Here's how the part is built. I have some questions about the finished solid (model axes, mm). A direction names the side the tool comes from. Round coordinates to 2 decimals unless told otherwise and drop trailing zeros. Loops run counter-clockwise (first coordinate to the right, second up) from the corner with the lowest first, then second, coordinate; pieces in that order, holes last. Notation, with made-up numbers: M 79.25,72.25 L 106.25,72.25 A34 cw 106.25,109.25 Z; hole C 12.25,55.5 d9. An arc over 180 degrees is marked long. Use a Markdown table: item, result.
from build123d import *

# Parameters (mm, degrees)
BODYS_W                        = 48
BODYS_H                        = 114
BODY_DEPTH                     = 1.7
MIRROR1_START                  = -1.7
MIRROR1_OUTLINE_R              = 4.1
MIRROR1_DEPTH                  = 3.4
KNUCKLEBODY_REACH              = 63.87
KNUCKLEBODY_DIRECTION_2_REACH  = 63.87
KNUCKLECUT_DEPTH               = 71.965414111
KNUCKLECUT_DEPTH_BACK          = 71.965414111
KNUCKLECUTS_W                  = 17
KNUCKLECUTS_H                  = 22
HOLECHAMFER_SIZE               = 1.4
F_11_0_11_DIAMETER_HOLE2_D     = 11
F_11_0_11_DIAMETER_HOLE2_DEPTH = 4
F_11_0_11_DIAMETER_HOLE2_TIP   = 3.304733405


# Read off the part's stored shape, not the designer's step: Mirror1
with BuildPart() as part:
    # BodyS → Body (new, symmetric)
    with BuildSketch(Plane.XY):
        Rectangle(BODYS_W, BODYS_H)
    extrude(amount=BODY_DEPTH, both=True)

    # Mirror1 outline → Mirror1 (cut)
    with BuildSketch(Plane.XY.offset(MIRROR1_START)):
        with Locations((-14.5, 15.5)):
            Circle(MIRROR1_OUTLINE_R)
        with Locations((1.5, 44)):
            Circle(MIRROR1_OUTLINE_R)
        with Locations((-14.5, -15.5)):
            Circle(MIRROR1_OUTLINE_R)
        with Locations((1.5, -44)):
            Circle(MIRROR1_OUTLINE_R)
    extrude(amount=MIRROR1_DEPTH, mode=Mode.SUBTRACT)

    # KnuckleBody: up to this face of the body (flat: up to its plane)
    knucklebody_end = Plane(part.part.faces().sort_by_distance((0, 57, 0))[0])
    # KnuckleBodyS → KnuckleBody (add, up to the picked face)
    with BuildSketch(Plane(origin=(0, 0, 0), x_dir=(1, 0, 0), z_dir=(0, 1, 0)), mode=Mode.PRIVATE) as knucklebody_sk1:
        with BuildLine():
            Line((25.386415094, -2.62754717), (28.555471698, -1.395849057))
            Line((28.555471698, -1.395849057), (29.678490566, -4.285283019))
            ThreePointArc((29.678490566, -4.285283019), (37.25246893, -4.451961541), (32.014716981, 1.021509434))
            Line((32.014716981, 1.021509434), (25.956226415, -1.333207547))
            ThreePointArc((25.956226415, -1.333207547), (24.995158089, -1.607509809), (24, -1.7))
            Line((24, -1.7), (24, 1.7))
            ThreePointArc((24, 1.7), (24.36857707, 1.734255626), (24.724528302, 1.835849057))
            Line((24.724528302, 1.835849057), (30.783018868, 4.190566038))
            ThreePointArc((30.783018868, 4.190566038), (40.364272432, -5.821880867), (26.509433962, -5.516981132))
            Line((26.509433962, -5.516981132), (25.386415094, -2.62754717))
        make_face()
    knucklebody_tool1 = split(extrude(knucklebody_sk1.sketch, amount=KNUCKLEBODY_REACH, mode=Mode.PRIVATE), bisect_by=knucklebody_end, keep=Keep.BOTH, mode=Mode.PRIVATE)
    add(knucklebody_tool1.solids().sort_by(Axis((26.159241, 0, 3.990133), (0, 1, 0)))[0])

    # KnuckleBody direction 2: up to this face of the body (flat: up to its plane)
    knucklebody_direction_2_end = Plane(part.part.faces().sort_by_distance((0, -57, 0))[0])
    # KnuckleBodyS → KnuckleBody direction 2 (add, up to the picked face)
    with BuildSketch(Plane(origin=(0, 0, 0), x_dir=(1, 0, 0), z_dir=(0, 1, 0)), mode=Mode.PRIVATE) as knucklebody_direction_2_sk1:
        with BuildLine():
            Line((25.386415094, -2.62754717), (28.555471698, -1.395849057))
            Line((28.555471698, -1.395849057), (29.678490566, -4.285283019))
            ThreePointArc((29.678490566, -4.285283019), (37.25246893, -4.451961541), (32.014716981, 1.021509434))
            Line((32.014716981, 1.021509434), (25.956226415, -1.333207547))
            ThreePointArc((25.956226415, -1.333207547), (24.995158089, -1.607509809), (24, -1.7))
            Line((24, -1.7), (24, 1.7))
            ThreePointArc((24, 1.7), (24.36857707, 1.734255626), (24.724528302, 1.835849057))
            Line((24.724528302, 1.835849057), (30.783018868, 4.190566038))
            ThreePointArc((30.783018868, 4.190566038), (40.364272432, -5.821880867), (26.509433962, -5.516981132))
            Line((26.509433962, -5.516981132), (25.386415094, -2.62754717))
        make_face()
    knucklebody_direction_2_tool1 = split(extrude(knucklebody_direction_2_sk1.sketch, amount=-KNUCKLEBODY_DIRECTION_2_REACH, mode=Mode.PRIVATE), bisect_by=knucklebody_direction_2_end, keep=Keep.BOTH, mode=Mode.PRIVATE)
    add(knucklebody_direction_2_tool1.solids().sort_by(Axis((26.159241, 0, 3.990133), (0, -1, 0)))[0])

    # KnuckleCutS → KnuckleCut (cut, two sides: drawn at the far end of the back side and taken through both)
    with BuildSketch(Plane.XY.offset(-KNUCKLECUT_DEPTH_BACK)):
        with Locations((32.5, 46)):
            Rectangle(KNUCKLECUTS_W, KNUCKLECUTS_H)
        with Locations((32.5, -46)):
            Rectangle(KNUCKLECUTS_W, KNUCKLECUTS_H)
        with Locations((32.5, 0)):
            Rectangle(KNUCKLECUTS_W, KNUCKLECUTS_H)
    extrude(amount=KNUCKLECUT_DEPTH + KNUCKLECUT_DEPTH_BACK, mode=Mode.SUBTRACT)

    # HoleChamfer
    holechamfer_edges = [part.edges().sort_by_distance(p)[0] for p in [
        (-18.6, 15.5, 1.7),
        (-2.6, 44, 1.7),
        (-18.6, -15.5, 1.7),
        (-2.6, -44, 1.7),
    ]]
    chamfer(holechamfer_edges, length=HOLECHAMFER_SIZE)

    # Ø11.0 (11) Diameter Hole2
    with Locations(Plane(origin=(0, -35, 0), x_dir=(-1, 0, 0), z_dir=(0, -1, 0))):
        with Locations((-33.5, -2.8)):
            Hole(F_11_0_11_DIAMETER_HOLE2_D / 2, depth=F_11_0_11_DIAMETER_HOLE2_DEPTH)
            with Locations((0, 0, -(F_11_0_11_DIAMETER_HOLE2_DEPTH + F_11_0_11_DIAMETER_HOLE2_TIP / 2))):  # 118° drill point
                Cone(0, F_11_0_11_DIAMETER_HOLE2_D / 2, F_11_0_11_DIAMETER_HOLE2_TIP, mode=Mode.SUBTRACT)


solid = part.part
1. I need wall thicknesses on probe 1 along Y at (x, z) = (1.5, -1.3); probe 2 along Y at (x, z) = (-14.5, -1); probe 3 along Z at (x, y) = (33.5, -32.15). Which ranges of each line are inside material? Lowest first, please. Write a range as from..to.
Answer sheet:
| item | result |
|---|---|
| probe 1 | -57..-48.1, -39.9..39.9, 48.1..57 |
| probe 2 | -57..-19.6, -11.4..11.4, 19.6..57 |
| probe 3 | -4.7..-2.7, 8.3..10.3 |
2. Imagine slicing it at D-D, the plane x = 12. Write out the boundary of the cut face in (y, z), then the cut area to 3 significant figures.
Answer sheet:
| item | result |
|---|---|
| outline | M -57,-1.7 L 57,-1.7 L 57,1.7 L -57,1.7 Z |
| area | 388 mm2 |
3. We'd pull the mould along Y, two halves only. Please class faces 5 (the face through (-17.754, 13.005, -0.714)), 6 (the face through (29, -35, -1)), 7 (the face through (30, 11, -1)), 8 (the face through (40.46, 23.17, 5.59)): +Y half, -Y half, draft (parallel to the pull), parting line (faces both ways), or undercut.
Answer sheet:
| item | result |
|---|---|
| face 5 | undercut |
| face 6 | -Y half |
| face 7 | undercut |
| face 8 | draft |
4. For pin 1 Ø4 at (x, y) = (25, -3.5) entering from +Z; pin 2 Ø13 at (x, y) = (1.5, 44) entering from -Z; pin 3 Ø4.5 at (x, z) = (33, 1.5) entering from -Y; pin 4 Ø1 at (y, z) = (-45, 0) entering from +X, each with a flat end and sliding along its axis, tell me the tip position at first contact or that it passes through.
Answer sheet:
| item | result |
|---|---|
| pin 1 | z = 1.7 |
| pin 2 | z = -1.7 |
| pin 3 | through |
| pin 4 | x = 24 |
5. Imagine slicing it at A-A, the plane y = -15.5. Write out the boundary of the cut face in (x, z).
Answer sheet:
| item | result |
|---|---|
| outline | M -24,-1.7 L -18.6,-1.7 L -18.6,0.3 L -20,1.7 L -24,1.7 Z; M -10.4,-1.7 L 24,-1.7 A2 cw 24.72,-1.84 L 30.78,-4.19 A7.5 ccw long 26.51,5.52 L 25.39,2.63 L 28.56,1.4 L 29.68,4.29 A4.1 cw long 32.01,-1.02 L 25.96,1.33 A5.4 ccw 24,1.7 L -9,1.7 L -10.4,0.3 Z |
6. Imagine slicing it at B-B, the plane x = -14.5. Write out the boundary of the cut face in (y, z).
Answer sheet:
| item | result |
|---|---|
| outline | M -57,-1.7 L -19.6,-1.7 L -19.6,0.3 L -21,1.7 L -57,1.7 Z; M -11.4,-1.7 L 11.4,-1.7 L 11.4,0.3 L 10,1.7 L -10,1.7 L -11.4,0.3 Z; M 19.6,-1.7 L 57,-1.7 L 57,1.7 L 21,1.7 L 19.6,0.3 Z |
7. Which directions (+Z, -Z, +X, -X, +Y, -Y) give clear straight access to the entire face, cutting with the end or side of a thin tool? Please do faces 1 (the face through (27, -23, 2)), 2 (the face through (24, 46, 0)), 3 (the face through (0, 1, -1.7)), 4 (the face through (24, 0, 0)).
Answer sheet:
| item | result |
|---|---|
| face 1 | +Y, -Y |
| face 2 | +Z, -Z, +X, +Y |
| face 3 | -Z, -X, +Y, -Y |
| face 4 | +Z, -Z, +X |
8. Imagine slicing it at C-C, the plane y = -33. Write out the boundary of the cut face in (x, z), then the cut area to 3 significant figures.
Answer sheet:
| item | result |
|---|---|
| outline | M -24,-1.7 L 24,-1.7 A2 cw 24.72,-1.84 L 30.78,-4.19 A7.5 ccw long 26.51,5.52 L 25.39,2.63 L 28.14,1.56 A5.5 cw long 28.6,0.31 L 25.96,1.33 A5.4 ccw 24,1.7 L -24,1.7 Z |
| area | 255 mm2 |
